For this review, use the dimensioned drawing (mm, ordinates from the lowest corner) and the shaded views. Round coordinates to 2 decimals unless told otherwise and drop trailing zeros. Loops run counter-clockwise (first coordinate to the right, second up) from the corner with the lowest first, then second, coordinate; pieces in that order, holes last. Notation, with made-up numbers: M 41.25,1.25 L 95.25,1.25 A25 cw 95.25,17.25 Z; hole C 46.5,60 d7. An arc over 180 degrees is marked long. One line per item, written item: value. Start each with the question number.
Item 1: We need section C-C (z = 57.5). State how many separate pieces and enclosed holes the cut face has, then the cut area to 3 significant figures.
Item 2: For line 1 along X through (y, z) = (23.5, 22) (1 decimal); line 2 along Y through (x, z) = (55.5, 15); line 3 along X through (y, z) = (25, 39), list the stretches that pass through material, from the lowest coordinate up.
Item 3: We need section A-A (y = 25.4). Write out the cut boundary in (x, z) (1 decimal), then the cut area to 3 significant figures.
Item 4: We need section B-B (x = 16). Write out the cut boundary in (y, z).
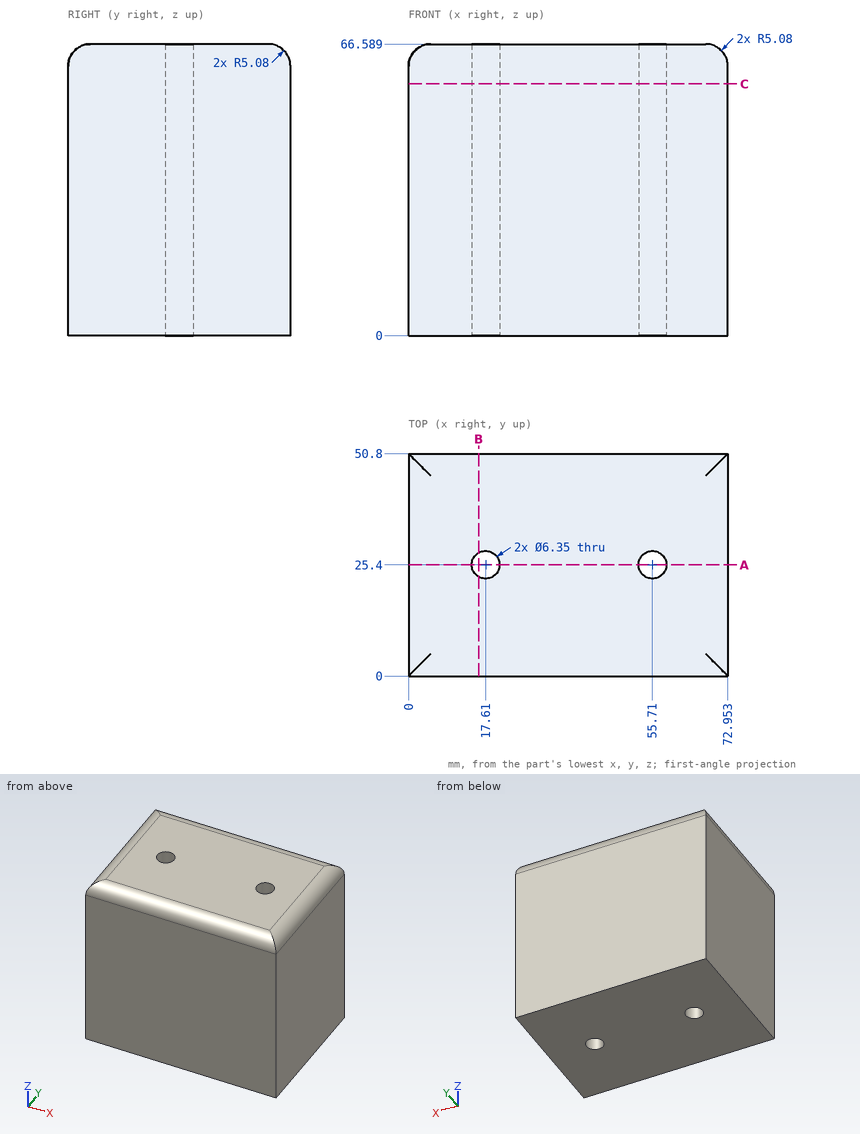
A:
1. separate pieces: 1
1. enclosed holes: 2
1. area: 3,640 mm2
2. line 1: 0 to 15.1, 20.2 to 53.2, 58.3 to 73
2. line 2: 0 to 22.23, 28.57 to 50.8
2. line 3: 0 to 14.46, 20.76 to 52.56, 58.86 to 72.95
3. outline: M 0,0 L 14.4,0 L 14.4,66.6 L 5.1,66.6 A5.1 ccw 0,61.5 Z; M 20.8,0 L 52.5,0 L 52.5,66.6 L 20.8,66.6 Z; M 58.9,0 L 73,0 L 73,61.5 A5.1 ccw 67.9,66.6 L 58.9,66.6 Z
3. area: 4,000 mm2
4. outline: M 0,0 L 22.66,0 L 22.66,66.59 L 5.08,66.59 A5.08 ccw 0,61.51 Z; M 28.14,0 L 50.8,0 L 50.8,61.51 A5.08 ccw 45.72,66.59 L 28.14,66.59 Z
